Can you work these out from the model? Positions are in its coordinate system, mm. A direction names the side the tool comes from. Coordinates: 2 decimals unless noted, no trailing zeros. Order: outer loops, then holes, each group sorted by start corner. A loop starts at its lowest first (then second) coordinate and runs counter-clockwise, first axis right, second up. Notation, with made-up numbers: (38.25, 85) -> (49.25, 85) arc R16 cw to (49.25, 89) -> close; hole circle Ø10 at (37.5, -19.75). An arc over 180 degrees is marked (long way). Answer in a Markdown table with one row per item. Add a question column.
1. Will these pins go through, and if not, where does the flat tip stop? pin 1 (1.5 mm diameter, centred on y = 0.5, z = -6.5, fed in from +X); pin 2 (10 mm diameter, centred on x = -29, y = -3, fed in from +Z); pin 3 (5 mm diameter, centred on x = -20.5, z = 6, fed in from -Y).
2. If I drill on line 1 along X through (y, z) = (-8.5, 3.25); line 2 along Z through (x, y) = (41, -1.5); line 3 along Y through (x, z) = (54.5, 0.25), over which ranges is the centre line in solid material (lowest first)? Write a range as [from, to].
3. On a 3-axis mill with a long thin cutter (end or side, diameter ignored), from which of +Z, -Z, +X, -X, +Y, -Y can I reach the whole of each face in a straight line? I mean faces 1 (the face through (-93.06, 4.96, 8.55)), 2 (the face through (-84.534, 0.2, -6.5)). Say none if no direction works.
4. Imagine slicing it at A-A on x = -72. Write out the boundary of the cut face in (y, z).
from build123d import *

# Parameters (mm, degrees)
SKETCH5_R           = 6.35
BOSS_EXTRUDE3_DEPTH = 177.8
CHAMFER1_SIZE       = 1.195753846
BOSS_EXTRUDE4_DEPTH = 8.73125
SKETCH8_OUTSIDE_W   = 708.434
SKETCH8_OUTSIDE_H   = 711.382
SKETCH8_OUTSIDE_R   = 9.525
CUT_EXTRUDE3_DEPTH  = 187.53125
CUT_EXTRUDE3_TAPER  = 60
CUT_EXTRUDE4_DEPTH  = 0.254
CIRPATTERN1_COUNT   = 3


with BuildPart() as part:
    # Sketch5 → Boss-Extrude3 (new body)
    with BuildSketch(Plane(origin=(93.265625, 0, 0), x_dir=(0, 0, -1), z_dir=(1, 0, 0))):
        Circle(SKETCH5_R)
    extrude(amount=-BOSS_EXTRUDE3_DEPTH)

    # Chamfer1
    chamfer1_edges = [part.edges().sort_by_distance(p)[0] for p in [
        (93.265625, 0, 6.35),
    ]]
    chamfer(chamfer1_edges, length=CHAMFER1_SIZE)

    # Sketch6 → Boss-Extrude4 (add)
    with BuildSketch(Plane.ZY.offset(84.534375)):
        Polygon((9.525, 5.499261314), (0, 10.998522628), (-9.525, 5.499261314), (-9.525, -5.499261314), (0, -10.998522628), (9.525, -5.499261314), align=None)
    extrude(amount=BOSS_EXTRUDE4_DEPTH)

    # Sketch8 outside → Cut-Extrude3 (cut, through all)
    with BuildSketch(Plane.ZY.offset(93.265625)):
        Rectangle(SKETCH8_OUTSIDE_W, SKETCH8_OUTSIDE_H)
        Circle(SKETCH8_OUTSIDE_R, mode=Mode.SUBTRACT)
    extrude(amount=-CUT_EXTRUDE3_DEPTH, taper=CUT_EXTRUDE3_TAPER, mode=Mode.SUBTRACT)

    # Sketch12 → Cut-Extrude4 (cut)
    with BuildSketch(Plane.ZY.offset(93.265625)):
        with BuildLine():
            Line((0.28575, 7.33425), (0.28575, 4.09575))
            ThreePointArc((0.28575, 4.09575), (0, 3.81), (-0.28575, 4.09575))
            Line((-0.28575, 4.09575), (-0.28575, 7.33425))
            ThreePointArc((-0.28575, 7.33425), (0, 7.62), (0.28575, 7.33425))
        make_face()
    cut_extrude4 = extrude(amount=-CUT_EXTRUDE4_DEPTH, mode=Mode.SUBTRACT)

    # CirPattern1: Cut-Extrude4 ×3 about axis
    cirpattern1_axis = Axis((0, 0, 0), (1, 0, 0))
    for i in range(1, CIRPATTERN1_COUNT):
        add(cut_extrude4.rotate(cirpattern1_axis, i * 360 / CIRPATTERN1_COUNT), mode=Mode.SUBTRACT)


solid = part.part
Answers follow:
| question | item | result |
|---|---|---|
| 1 | pin 1 | stops at x = 92.65 |
| 1 | pin 2 | stops at z = 6.35 |
| 1 | pin 3 | stops at y = -5.3 |
| 2 | line 1 | x = [-93.27, -84.53] |
| 2 | line 2 | z = [-6.17, 6.17] |
| 2 | line 3 | y = [-6.35, 6.35] |
| 3 | face 1 | +Z, -X, +Y |
| 3 | face 2 | +X |
| 4 | outline | circle Ø12.7 at (0, 0) |
